```python
from build123d import *

# Parameters (mm, degrees)
F0_R     = 4.5
F1_DEPTH = 1.5
F0_W     = 2
F0_H     = 4.459151
F2_DEPTH = 5
F3_DEPTH = 6
F4_R     = 1.15
F5_DEPTH = 25


with BuildPart() as f1:
    # F0 (on Top) → F1 (new body)
    with BuildSketch(Plane.XY):
        with BuildLine():
            ThreePointArc((-7.173268, 1.602102), (-0.80591, -7.305683), (7.35, 0))
            ThreePointArc((7.35, 0), (7.305683, 0.80591), (7.173268, 1.602102))
            ThreePointArc((7.173268, 1.602102), (0, 7.35), (-7.173268, 1.602102))
        make_face()
        Circle(F0_R, mode=Mode.SUBTRACT)
    extrude(amount=F1_DEPTH)

    # F0 (on Top) → F2 (join)
    with BuildSketch(Plane.XY):
        Polygon((-9.510325, 9), (-7, 9), (-7, 12.338503), (-9, 12.338503), (-9.510325, 12.338503), align=None)
        with BuildLine():
            Line((-9.510325, 6.091482), (-8.334513, 4.012281))
            ThreePointArc((-8.334513, 4.012281), (-5.798901, 7.206612), (-2.136001, 9))
            Line((-2.136001, 9), (-7, 9))
            Line((-7, 9), (-9.510325, 9))
            Line((-9.510325, 9), (-9.510325, 6.091482))
        make_face()
        with BuildLine():
            ThreePointArc((-7.173268, 1.602102), (0, 7.35), (7.173268, 1.602102))
            Line((7.173268, 1.602102), (8.334513, 4.012281))
            ThreePointArc((8.334513, 4.012281), (5.798901, 7.206612), (2.136001, 9))
            Line((2.136001, 9), (0, 9))
            Line((0, 9), (-2.136001, 9))
            ThreePointArc((-2.136001, 9), (-5.798901, 7.206612), (-8.334513, 4.012281))
            Line((-8.334513, 4.012281), (-7.173268, 1.602102))
        make_face()
        with BuildLine():
            Line((0, 9), (2.136001, 9))
            ThreePointArc((2.136001, 9), (1.075291, 9.187287), (0, 9.25))
            Line((0, 9.25), (0, 9))
        make_face()
        Polygon((7, 12.338503), (7, 9), (9.510325, 9), (9.510325, 12.338503), (9, 12.338503), align=None)
        with Locations((-8, 14.568078)):
            Rectangle(F0_W, F0_H)
        with Locations((8, 14.568078)):
            Rectangle(F0_W, F0_H)
        with BuildLine():
            ThreePointArc((2.136001, 9), (5.798901, 7.206612), (8.334513, 4.012281))
            Line((8.334513, 4.012281), (9.510325, 6.091482))
            Line((9.510325, 6.091482), (9.510325, 9))
            Line((9.510325, 9), (7, 9))
            Line((7, 9), (2.136001, 9))
        make_face()
    extrude(amount=F2_DEPTH)

    # F0 (on Top) → F3 (join)
    with BuildSketch(Plane.XY):
        with BuildLine():
            ThreePointArc((7.173268, 1.602102), (7.305683, 0.80591), (7.35, 0))
            ThreePointArc((7.35, 0), (-0.80591, -7.305683), (-7.173268, 1.602102))
            Line((-7.173268, 1.602102), (-8.334513, 4.012281))
            ThreePointArc((-8.334513, 4.012281), (-2.0577, -9.018224), (9.25, 0))
            ThreePointArc((9.25, 0), (9.018224, 2.0577), (8.334513, 4.012281))
            Line((8.334513, 4.012281), (7.173268, 1.602102))
        make_face()
    extrude(amount=F3_DEPTH)

    # F4 (on face) → F5 (cut)
    with BuildSketch(Plane(origin=(-9, 0, 0), x_dir=(0, -1, 0), z_dir=(-1, 0, 0))):
        with Locations((-14.394956, 2.5)):
            Circle(F4_R)
    extrude(amount=-F5_DEPTH, mode=Mode.SUBTRACT)


solid = f1.part
```
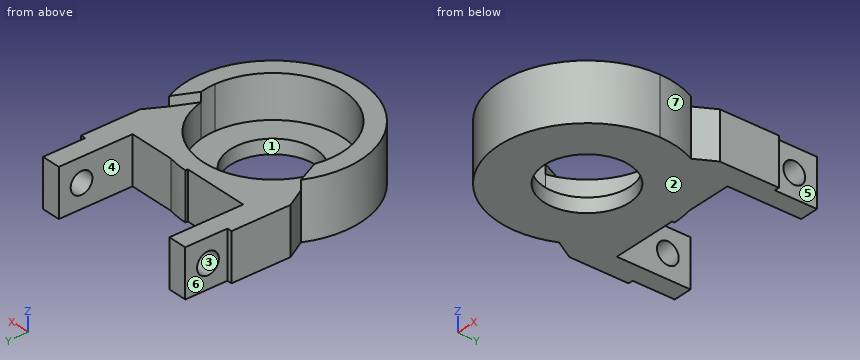
Source: CAD feature listing. Evaluate the final solid. Frame: model axes, mm. Face numbers are marked on the shaded views. A direction names the side the tool comes from. Coordinates: 2 decimals unless noted, no trailing zeros. Loops run counter-clockwise (first coordinate to the right, second up) from the corner with the lowest first, then second, coordinate; pieces in that order, holes last. Notation, with made-up numbers: M 15.5,79 L 29.5,79 A20 cw 29.5,91 Z; hole C -30.75,13 d2. An arc over 180 degrees is marked long. Put each result on its own line as item: value. Start each with the question number.
1) Cut plane B-B on y = -2. Return the cut outline in (x, z).
2) Cut plane A-A on z = 2.5. Return the cut outline in (x, y), then the cut area to 3 significant figures.
3) Cut plane C-C on z = 0.7. Return the cut outline in (x, y).
4) Cut plane D-D on x = -8. Return the cut outline in (y, z).
5) Pull-direction query (Z, two-part tool) for the marked faces 1, 2 and 3; classes: pulls with the +Z half, pulls with the -Z half, needs draft (parallel to the pull), parting line crosses it, or undercut.
6) Reachability of the marked faces 4, 5, 6 and 7 from +Z, -Z, +X, -X, +Y, -Y: full face, straight path, thin tool, end or side. Return the list, or none.
7) Contact query for flat-ended pins moving along their axis: pin 1 Ø2.5 at (y, z) = (14.39, 2.5) entering from +X; pin 2 Ø1.5 at (y, z) = (-2.5, 2.5) entering from -X; pin 3 Ø1.5 at (y, z) = (-1.5, 2) entering from -X. Output: stop coordinate, or through.
8) Ray query, L1, parallel to X at y = 0, z = 3.15; L2, parallel to Z at x = -0.25, y = 6.25; L3, parallel to Y at x = 8.5, z = 0.4. Return the intervals inside material, ascending. Write a range as from..to.
The answers:
1. outline: M -9.03,0 L -4.03,0 L -4.03,1.5 L -7.07,1.5 L -7.07,6 L -9.03,6 Z; M 4.03,0 L 9.03,0 L 9.03,6 L 7.07,6 L 7.07,1.5 L 4.03,1.5 Z
2. outline: M -9.51,6.09 L -8.33,4.01 A9.25 ccw long 9.25,0 A9.25 ccw 8.33,4.01 L 9.51,6.09 L 9.51,12.34 L 9,12.34 L 9,13.24 L 7,13.24 L 7,9 L 2.14,9 A9.25 ccw 0,9.25 L 0,9 L -7,9 L -7,13.24 L -9,13.24 L -9,12.34 L -9.51,12.34 Z; M -9,15.54 L -7,15.54 L -7,16.8 L -9,16.8 Z; M 7,15.54 L 9,15.54 L 9,16.8 L 7,16.8 Z; hole M 7.17,1.6 A7.35 ccw long 7.35,0 A7.35 ccw Z
2. area: 155 mm²
3. outline: M -9.51,6.09 L -8.33,4.01 A9.25 ccw long 9.25,0 A9.25 ccw 8.33,4.01 L 9.51,6.09 L 9.51,12.34 L 9,12.34 L 9,16.8 L 7,16.8 L 7,9 L 2.14,9 A9.25 ccw 0,9.25 L 0,9 L -7,9 L -7,16.8 L -9,16.8 L -9,12.34 L -9.51,12.34 Z; hole C 0,0 d9
4. outline: M -4.64,0 L 16.8,0 L 16.8,5 L 3.32,5 L 3.32,6 L -4.64,6 Z; hole C 14.39,2.5 d2.3
5. face 1: needs draft
5. face 2: pulls with the -Z half
5. face 3: undercut
6. face 4: +Z, -Z, +Y
6. face 5: +Z, -Z, +X, +Y
6. face 6: +Z, -Z, -X, +Y
6. face 7: +Z, -Z, +X
7. pin 1: stops at x = 9
7. pin 2: stops at x = -9.08
7. pin 3: stops at x = -9.22
8. L1: x = -9.25..-7.35, 7.35..9.25
8. L2: z = 0..1.5
8. L3: y = -3.65..3.65, 4.3..16.8
